Input: part model. Units: mm. Frame: model coordinates. Face numbers are marked on the shaded views. Coordinates: 2 decimals unless noted, no trailing zeros. Write each loop counter-clockwise with the first axis right and the second up, starting at its lowest first coordinate (ties: lowest second). Pieces come first, ordered by that corner, then holes.
1) Draft query along X for the marked faces 1, 2, 3 and 4. Return one class per face: pulls with the +X half, pulls with the -X half, needs draft (parallel to the pull), parting line crosses it, or undercut.
2) Section query C-C (z = 0.35). Output: boundary loops of the cut face in (x, y).
3) Line query: L1, parallel to Y at x = 3, z = 1.2; L2, parallel to X at y = 25, z = 0.95; L3, parallel to Y at x = 4.2, z = 0.3. Output: solid intervals per line, ascending.
4) Section query D-D (x = 1.75). Output: boundary loops of the cut face in (y, z), then the cut area to 3 significant figures.
5) Section query B-B (y = 5). Output: boundary loops of the cut face in (x, z), then the cut area to 3 significant figures.
6) Section query A-A (x = 3). Output: boundary loops of the cut face in (y, z).
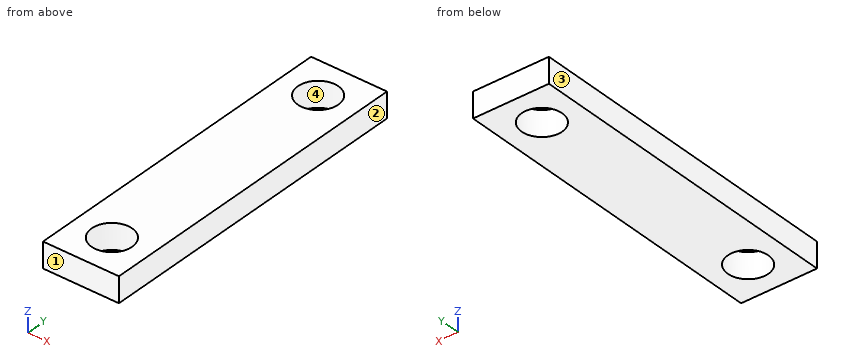
Autodesk Inventor part; units mm, degrees
ref_plane "YZ Plane" through (0, 0, 0) normal (1, 0, 0) x (0, 1, 0)
ref_plane "XZ Plane" through (0, 0, 0) normal (0, 1, 0) x (-1, 0, 0)
ref_plane "XY Plane" through (0, 0, 0) normal (0, 0, 1) x (1, 0, 0)
sketch "スケッチ1" plane through (0, 0, 0) normal (0, 0, 1) x (1, 0, 0)
  line L0 (0, 0) -> (6, 0)
  line L1 (6, 0) -> (6, 30)
  line L2 (6, 30) -> (0, 30)
  line L3 (0, 30) -> (0, 0)
  dimension "d0" = 6
  dimension "d1" = 30
extrude "押し出し1" add sketch "スケッチ1" along normal blind 2
sketch "スケッチ2" plane through (0, 0, 2) normal (0, 0, 1) x (1, 0, 0)
  line L0 (6, 30) -> (0, 30)
  line L1 (6, 0) -> (6, 30)
  line L2 (0, 0) -> (6, 0)
  point P0 (3, 25)
  point P1 (3, 5)
  dimension "d4" = 5
  dimension "d5" = 3
  dimension "d6" = 3
  dimension "d7" = 5
hole "穴1" at (3, 25, 2) at (3, 5, 2) direction (0, 0, -1) diameter 3.2 end through all
sketch "スケッチ4" plane through (0, 0, 2) normal (0, 0, 1) x (1, 0, 0)
  line L0 (6, 30) -> (0, 30)
  line L1 (6, 0) -> (6, 30)
  line L2 (0, 30) -> (6, 30)
  line L3 (6, 30) -> (6, 28)
  line L4 (6, 28) -> (0, 28)
  line L5 (0, 28) -> (0, 30)
  line L6 (0, 30) -> (0, 0)
  line L7 (0, 2) -> (6, 2)
  line L8 (6, 2) -> (6, 0)
  line L9 (6, 0) -> (0, 0)
  line L10 (0, 0) -> (0, 2)
  dimension "d18" = 2
  dimension "d19" = 2
extrude "押し出し2" cut sketch "スケッチ4" against normal blind 10 contours L1 L4 L5 L0 | L1 L9 L6 L7
properties part number "リンク30×6×2"
Answer:
1. face 1: needs draft
1. face 2: pulls with the +X half
1. face 3: pulls with the -X half
1. face 4: undercut
2. outline: (0, 2) - (6, 2) - (6, 28) - (0, 28) - close; hole circle Ø3.2 at (3, 5); hole circle Ø3.2 at (3, 25)
3. L1: y = 2 to 3.4, 6.6 to 23.4, 26.6 to 28
3. L2: x = 0 to 1.4, 4.6 to 6
3. L3: y = 2 to 3.94, 6.06 to 23.94, 26.06 to 28
4. outline: (2, 0) - (4, 0) - (4, 2) - (2, 2) - close; (6, 0) - (24, 0) - (24, 2) - (6, 2) - close; (26, 0) - (28, 0) - (28, 2) - (26, 2) - close
4. area: 44.0 mm2
5. outline: (0, 0) - (1.4, 0) - (1.4, 2) - (0, 2) - close; (4.6, 0) - (6, 0) - (6, 2) - (4.6, 2) - close
5. area: 5.60 mm2
6. outline: (2, 0) - (3.4, 0) - (3.4, 2) - (2, 2) - close; (6.6, 0) - (23.4, 0) - (23.4, 2) - (6.6, 2) - close; (26.6, 0) - (28, 0) - (28, 2) - (26.6, 2) - close
